from build123d import *

# Parameters (mm, degrees)
F1_DEPTH = 4.9
F2_SIZE  = 2
F3_SIZE  = 2


with BuildPart() as f1:
    # F0 (on Top) → F1 (new body)
    with BuildSketch(Plane.XY):
        Polygon((0, 0), (0, 9.55), (1.2, 9.55), (1.2, 8.35), (4.5, 9.9), (4.5, 11.5), (0, 11.5), (0, 12.5), (4.5, 12.5), (4.5, 14.1), (1.2, 15.65), (1.2, 14.45), (0, 14.45), (0, 17.6), (1.2, 17.6), (1.2, 16.4), (4.5, 17.95), (4.5, 19.55), (0, 19.55), (0, 20.55), (4.5, 20.55), (4.5, 22.15), (1.2, 23.7), (1.2, 22.5), (0, 22.5), (-2, 22.5), (-2, 2), (-12, 2), (-12, 21), (-10, 23), (-12, 25), (-14, 25), (-14, 0), align=None)
    extrude(amount=F1_DEPTH)

    # F2
    f2_edges = [f1.edges().sort_by_distance(p)[0] for p in [
        (-2, 2, 2.45),
    ]]
    chamfer(f2_edges, length=F2_SIZE)

    # F3
    f3_edges = [f1.edges().sort_by_distance(p)[0] for p in [
        (-12, 2, 2.45),
    ]]
    chamfer(f3_edges, length=F3_SIZE)


solid = f1.part
Geometry check sheet. Reference: the model listing, model coordinates, mm. A direction names the side the tool comes from. Round coordinates to 2 decimals unless told otherwise and drop trailing zeros. Order: outer loops, then holes, each group sorted by start corner. A loop starts at its lowest first (then second) coordinate and runs counter-clockwise, first axis right, second up. Notation, with made-up numbers: M 57,-39 L 103,-39 A12 ccw 103,-18 Z; hole C 26,-29.75 d11. An arc over 180 degrees is marked long. Write each question's results on one line, items separated by ' | '. Start each with the question number.
1. Cross-section at D-D on x = -5.5. Record the boundary of the cut face in (y, z), plus the area to 3 significant figures.
2. Cross-section at C-C on x = 2.5. Record the boundary of the cut face in (y, z), plus the area to 3 significant figures.
3. Material ranges on L1, parallel to Y at x = 0.5, z = 0.4; L2, parallel to X at y = 5.5, z = 2.65; L3, parallel to Y at x = 3.25, z = 4.6, recorded low to high. Write a range as from..to.
4. Go/stop test with flat-tipped pins: P1, Ø1.3, axis at x = 1, z = 3, coming from the -Y side; P2, Ø2.5, axis at x = -1, z = 2.5, coming from the +Y side; P3, Ø10, axis at x = 1, y = 15.5, coming from the -Z side; P4, Ø0.5, axis at y = 20, z = 2.5, coming from the +X side. Record where each tip stops, or that it passes through.
5. Draft check along Y on faces 4 (the face through (-3, 3, 2)), 5 (the face through (1.2, 23, 2)), 6 (the face through (0, 16, 2)). Enter one of: pulls with the +Y half, pulls with the -Y half, needs draft (parallel to the pull), parting line crosses it, or undercut.
6. Cross-section at A-A on y = 5. Record the boundary of the cut face in (x, z).
7. Set-up check for faces 1 (the face through (-11, 3, 2)), 2 (the face through (0, 22.5, 2)), 3 (the face through (2, 20.55, 2)): record each of +Z, -Z, +X, -X, +Y, -Y from which the full face is reachable in a straight line by a thin tool's end or side.
Resolved:
1) outline: M 0,0 L 2,0 L 2,4.9 L 0,4.9 Z | area: 9.80 mm2
2) outline: M 8.96,0 L 11.5,0 L 11.5,4.9 L 8.96,4.9 Z; M 12.5,0 L 15.04,0 L 15.04,4.9 L 12.5,4.9 Z; M 17.01,0 L 19.55,0 L 19.55,4.9 L 17.01,4.9 Z; M 20.55,0 L 23.09,0 L 23.09,4.9 L 20.55,4.9 Z | area: 49.8 mm2
3) L1: 9.55..11.5, 12.5..14.45, 17.6..19.55, 20.55..22.5 | L2: -14..-12, -2..0 | L3: 9.31..11.5, 12.5..14.69, 17.36..19.55, 20.55..22.74
4) P1: y = 8.35 | P2: y = 22.5 | P3: z = 0 | P4: x = 0
5) face 4: pulls with the +Y half | face 5: needs draft | face 6: undercut
6) outline: M -14,0 L -12,0 L -12,4.9 L -14,4.9 Z; M -2,0 L 0,0 L 0,4.9 L -2,4.9 Z
7) face 1: +Z, -Z | face 2: +Z, -Z, +Y | face 3: +Z, -Z, +X
